```python
from build123d import *

# Parameters (mm, degrees)
F1_DEPTH      = 25
F1_DEPTH_BACK = 25
F2_R          = 4.99999


# Not quite as in the source:
# - a fillet or chamfer is up to 0.001 mm smaller than in the source, because OpenCascade refuses the exact size


with BuildPart() as f1:
    # F0 (on Top) → F1 (new body, two sides)
    with BuildSketch(Plane.XY) as f1_sk:
        Polygon((30, 15), (-30, 15), (-30, -15), (-25, -15), (-25, 10), (25, 10), (25, -15), (30, -15), align=None)
    extrude(amount=F1_DEPTH)
    extrude(f1_sk.sketch, amount=-F1_DEPTH_BACK)

    # F2 (radius 5 in the source; OpenCascade refuses exactly that, so slightly less here)
    f2_edges = [f1.edges().sort_by_distance(p)[0] for p in [
        (-30, 15, 0),
        (30, 15, 0),
        (30, -15, 0),
        (-30, -15, 0),
    ]]
    fillet(f2_edges, radius=F2_R)


solid = f1.part
```
Input: part model. Units: mm. Frame: model coordinates. A direction names the side the tool comes from. Coordinates: 2 decimals unless noted, no trailing zeros. Loops run counter-clockwise (first coordinate to the right, second up) from the corner with the lowest first, then second, coordinate; pieces in that order, holes last. Notation, with made-up numbers: M 87.25,-26 L 144.25,-26 A17 cw 144.25,6 Z; hole C 77,56.25 d2. An arc over 180 degrees is marked long. Use a Markdown table: item, result. Add a question column.
1) Section D-D, the plane x = 5.5. Return the cut outline in (y, z), plus the area to 3 significant figures.
2) Section C-C, the plane y = -11.5. Return the cut outline in (x, z), plus the area to 3 significant figures.
3) Pin query (flat end, axial travel): P1, Ø15, axis at x = 12.5, z = -1.5, coming from the -Y side. Return the tip coordinate at first contact, or that it passes through.
4) Section A-A, the plane y = -7.5. Return the cut outline in (x, z).
5) Set-up query: faces 5 (the flat face through (-25, -3, 0)), 6 (the cylindrical face through (-28, 14, 0)). Return all of +Z, -Z, +X, -X, +Y, -Y with unobstructed straight access to the full face (end or side cutting, diameter ignored); none if empty.
6) Draft query along X for faces 1 (the flat face through (0, 10, 0)), 2 (the flat face through (-30, 0, 0)), 3 (the flat face through (-0.4, 10.2, 25)), 4 (the cylindrical face through (29, -13, 0)). Return one class per face: +X half, -X half, draft (parallel to the pull), parting line (faces both ways), or undercut.
7) Line query: L1, parallel to X at y = 8.5, z = 2; L2, parallel to Y at x = -3, z = 22; L3, parallel to X at y = 10.25, z = -9. Output: solid intervals per line, ascending. Write a range as from..to.
Answer below:
| question | item | result |
|---|---|---|
| 1 | outline | M 10,-25 L 15,-25 L 15,25 L 10,25 Z |
| 1 | area | 250 mm2 |
| 2 | outline | M -29.77,-25 L -25,-25 L -25,25 L -29.77,25 Z; M 25,-25 L 29.77,-25 L 29.77,25 L 25,25 Z |
| 2 | area | 477 mm2 |
| 3 | P1 | y = 10 |
| 4 | outline | M -30,-25 L -25,-25 L -25,25 L -30,25 Z; M 25,-25 L 30,-25 L 30,25 L 25,25 Z |
| 5 | face 5 | +Z, -Z, -Y |
| 5 | face 6 | +Z, -Z, -X, +Y |
| 6 | face 1 | undercut |
| 6 | face 2 | -X half |
| 6 | face 3 | draft |
| 6 | face 4 | +X half |
| 7 | L1 | -30..-25, 25..30 |
| 7 | L2 | 10..15 |
| 7 | L3 | -29.99..29.99 |
